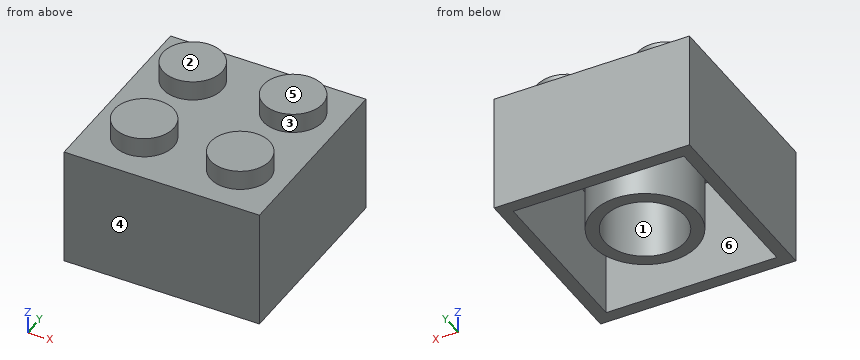
from build123d import *

# Parameters (mm, degrees)
F0_W          = 15.8
F0_H          = 15.8
F1_DEPTH      = 9.6
F4_R          = 2.4
F6_DEPTH      = 1.6
F5_R          = 2.4
F7_DEPTH      = 1.6
F3_R          = 2.4
F8_DEPTH      = 1.6
F2_R          = 2.4
F9_DEPTH      = 1.6
F10_T         = -1
F11_R         = 4.255
F12_DEPTH     = 8.13
F13_T         = 1
F13_T3_DEPTH  = 10.6
F13_T5_DEPTH  = 15.8
F13_T7_DEPTH  = 15.8
F13_T18_ANGLE = 35.7281901551
F13_T20_ANGLE = 210.9230732258
F13_T22_ANGLE = 74.818128958
F13_T24_ANGLE = 41.9866867229
F13_T28_ANGLE = 82.2344866513


# Not quite as in the source:
# - a shell that OpenCascade refuses in one call is made with other operations: the cavity is built on its own and cut out


with BuildPart() as f1:
    # F0 (on Top) → F1 (new body)
    with BuildSketch(Plane.XY):
        Rectangle(F0_W, F0_H)
    extrude(amount=-F1_DEPTH)

    # F4 (on face) → F6 (join)
    with BuildSketch(Plane.XY):
        with Locations((-3.7834926043, -3.5802270286)):
            Circle(F4_R)
    extrude(amount=F6_DEPTH)

    # F5 (on face) → F7 (join)
    with BuildSketch(Plane.XY):
        with Locations((4.0790652856, -3.737478517)):
            Circle(F5_R)
    extrude(amount=F7_DEPTH)

    # F3 (on face) → F8 (join)
    with BuildSketch(Plane.XY):
        with Locations((4.1130073369, 4.042240791)):
            Circle(F3_R)
    extrude(amount=F8_DEPTH)

    # F2 (on face) + F3 (on face) → F9 (join)
    with BuildSketch(Plane.XY):
        with Locations((-4.0000770241, 4.039389547)):
            Circle(F2_R)
    with BuildSketch(Plane.XY):
        with Locations((4.1130073369, 4.042240791)):
            Circle(F3_R)
    extrude(amount=F9_DEPTH)

    # F10
    f10_openings = [f1.faces().sort_by_distance(p)[0] for p in [
        (0, 0, -9.6),
    ]]
    offset(amount=F10_T, openings=f10_openings, kind=Kind.INTERSECTION)

    # F11 (on face) → F12 (join)
    with BuildSketch(Plane(origin=(0, 0, -1), x_dir=(1, 0, 0), z_dir=(0, 0, -1))):
        Circle(F11_R)
    extrude(amount=F12_DEPTH)

    # F13: shell of thickness 1, made by hand


with BuildPart() as f13_core1:
    # F13_t2: copy of F1
    add(f1.part)

    # the walls: a layer under each face that stays
    f13_faces = [f13_core1.faces().sort_by_distance(p)[0] for p in [
        (7.9, 0, -4.8),
        (0, -7.9, -4.8),
        (0, 7.9, -4.8),
        (0, 0, 0),
        (-7.3733333333, -7.3733333333, -9.6),
        (-7.9, 0, -4.8),
        (-6.1834926043, -3.5802270286, 0.8),
        (1.6790652856, -3.737478517, 0.8),
        (-6.4000770241, 4.039389547, 0.8),
        (1.7130073369, 4.042240791, 0.8),
        (6.9, 0, -5.3),
        (0, -6.9, -5.3),
        (-6.9, 0, -5.3),
        (0, 6.9, -5.3),
        (-3.7834926043, -3.5802270286, 1.6),
        (4.0790652856, -3.737478517, 1.6),
        (-4.0000770241, 4.039389547, 1.6),
        (4.1130073369, 4.042240791, 1.6),
        (-4.6, 0, -1),
        (2.6790652856, -3.737478517, -0.2),
        (-4.255, 0, -5.065),
        (-5.1834926043, -3.5802270286, -0.2),
        (-5.4000770241, 4.039389547, -0.2),
        (2.7130073369, 4.042240791, -0.2),
        (3.1153566982, -2.8544722668, -1),
        (4.0790652856, -3.737478517, 0.6),
        (-3.0174039644, -2.8552959816, -1),
        (-3.7834926043, -3.5802270286, 0.6),
        (-4.0000770241, 4.039389547, 0.6),
        (4.1130073369, 4.042240791, 0.6),
    ]]
    thicken(f13_faces, amount=-F13_T, mode=Mode.SUBTRACT)

    # F13_s4 → F13_t3 (cut)
    with BuildSketch(Plane.XY.offset(-10.6)):
        Polygon((6.89, -6.89), (7.9, -6.9), (7.9, -7.9), (6.9, -7.9), align=None)
        Polygon((6.89, 6.89), (7.9, 6.9), (7.9, 7.9), (6.9, 7.9), align=None)
        Polygon((-6.89, -6.89), (-6.9, -7.9), (-7.9, -7.9), (-7.9, -6.9), align=None)
        Polygon((-6.89, 6.89), (-7.9, 6.9), (-7.9, 7.9), (-6.9, 7.9), align=None)
    extrude(amount=F13_T3_DEPTH, mode=Mode.SUBTRACT)

    # F13_s6 → F13_t5 (cut)
    with BuildSketch(Plane.XZ.offset(-7.9)):
        Polygon((6.89, -1.01), (7.9, -1), (7.9, 0), (6.9, 0), align=None)
        Polygon((-6.89, -1.01), (-7.9, -1), (-7.9, 0), (-6.9, 0), align=None)
    extrude(amount=F13_T5_DEPTH, mode=Mode.SUBTRACT)

    # F13_s8 → F13_t7 (cut)
    with BuildSketch(Plane.YZ.offset(-7.9)):
        Polygon((-6.89, -1.01), (-7.9, -1), (-7.9, 0), (-6.9, 0), align=None)
        Polygon((6.89, -1.01), (7.9, -1), (7.9, 0), (6.9, 0), align=None)
    extrude(amount=F13_T7_DEPTH, mode=Mode.SUBTRACT)

    # F13_s9 → F13_t10 (revolve, cut)
    with BuildSketch(Plane.XZ.offset(3.5802270286)):
        Polygon((-1.3734926043, 0.01), (-1.3834926043, -1), (-2.3834926043, -1), (-2.3834926043, 0), align=None)
    revolve(axis=Axis((-3.7834926043, -3.5802270286, 0), (0, 0, 1)), mode=Mode.SUBTRACT)

    # F13_s11 → F13_t12 (revolve, cut)
    with BuildSketch(Plane.XZ.offset(3.737478517)):
        Polygon((6.4890652856, 0.01), (6.4790652856, -1), (5.4790652856, -1), (5.4790652856, 0), align=None)
    revolve(axis=Axis((4.0790652856, -3.737478517, 0), (0, 0, 1)), mode=Mode.SUBTRACT)

    # F13_s13 → F13_t14 (revolve, cut)
    with BuildSketch(Plane.XZ.offset(-4.039389547)):
        Polygon((-1.5900770241, 0.01), (-1.6000770241, -1), (-2.6000770241, -1), (-2.6000770241, 0), align=None)
    revolve(axis=Axis((-4.0000770241, 4.039389547, 0), (0, 0, 1)), mode=Mode.SUBTRACT)

    # F13_s15 → F13_t16 (revolve, cut)
    with BuildSketch(Plane.XZ.offset(-4.042240791)):
        Polygon((6.5230073369, 0.01), (6.5130073369, -1), (5.5130073369, -1), (5.5130073369, 0), align=None)
    revolve(axis=Axis((4.1130073369, 4.042240791, 0), (0, 0, 1)), mode=Mode.SUBTRACT)

    # F13_s17 → F13_t18 (revolve, cut)
    with BuildSketch(Plane.XZ):
        Polygon((4.265, -1.01), (4.255, 0), (3.255, 0), (3.255, -1), align=None)
    revolve(axis=Axis((0, 0, -1), (0, 0, -1)), revolution_arc=F13_T18_ANGLE, mode=Mode.SUBTRACT)

    # F13_s19 → F13_t20 (revolve, cut)
    with BuildSketch(Plane(origin=(0, 0, 0), x_dir=(0, 0, 1), z_dir=(0.5138867564, -0.8578580312, 0))):
        Polygon((-1.01, 4.265), (0, 4.255), (0, 3.255), (-1, 3.255), align=None)
    revolve(axis=Axis((0, 0, -1), (0, 0, -1)), revolution_arc=F13_T20_ANGLE, mode=Mode.SUBTRACT)

    # F13_s21 → F13_t22 (revolve, cut)
    with BuildSketch(Plane(origin=(0, 0, 0), x_dir=(0, 0, 1), z_dir=(0.7577618984, 0.6525311528, 0))):
        Polygon((-1.01, 4.265), (0, 4.255), (0, 3.255), (-1, 3.255), align=None)
    revolve(axis=Axis((0, 0, -1), (0, 0, -1)), revolution_arc=F13_T22_ANGLE, mode=Mode.SUBTRACT)

    # F13_s23 → F13_t24 (revolve, cut)
    with BuildSketch(Plane(origin=(-0.7265604619, -1.8440663308, 0), x_dir=(0, 0, 1), z_dir=(-0.3665725996, -0.9303894503, 0))):
        Polygon((-0.99, -3.7751765248), (-1, -2.7651765248), (-2, -2.7651765248), (-2, -3.7651765248), align=None)
    revolve(axis=Axis((4.0790652856, -3.737478517, -1), (0, 0, -1)), revolution_arc=F13_T24_ANGLE, mode=Mode.SUBTRACT)

    # F13_s25 → F13_t26 (revolve, cut)
    with BuildSketch(Plane.XZ.offset(3.737478517)):
        Polygon((5.4690652856, 0.59), (6.4790652856, 0.6), (6.4790652856, 1.6), (5.4790652856, 1.6), align=None)
    revolve(axis=Axis((4.0790652856, -3.737478517, 0.6), (0, 0, -1)), mode=Mode.SUBTRACT)

    # F13_s27 → F13_t28 (revolve, cut)
    with BuildSketch(Plane(origin=(-3.4098320419, 0.3261629687, 0), x_dir=(0, 0, 1), z_dir=(-0.9954563431, 0.0952190583, 0))):
        Polygon((-0.99, -2.5342203081), (-1, -1.5242203081), (-2, -1.5242203081), (-2, -2.5242203081), align=None)
    revolve(axis=Axis((-3.7834926043, -3.5802270286, -1), (0, 0, -1)), revolution_arc=F13_T28_ANGLE, mode=Mode.SUBTRACT)

    # F13_s29 → F13_t30 (revolve, cut)
    with BuildSketch(Plane.XZ.offset(3.5802270286)):
        Polygon((-2.3934926043, 0.59), (-1.3834926043, 0.6), (-1.3834926043, 1.6), (-2.3834926043, 1.6), align=None)
    revolve(axis=Axis((-3.7834926043, -3.5802270286, 0.6), (0, 0, -1)), mode=Mode.SUBTRACT)

    # F13_s31 → F13_t32 (revolve, cut)
    with BuildSketch(Plane.XZ.offset(-4.039389547)):
        Polygon((-2.6100770241, 0.59), (-1.6000770241, 0.6), (-1.6000770241, 1.6), (-2.6000770241, 1.6), align=None)
    revolve(axis=Axis((-4.0000770241, 4.039389547, 0.6), (0, 0, -1)), mode=Mode.SUBTRACT)

    # F13_s33 → F13_t34 (revolve, cut)
    with BuildSketch(Plane.XZ.offset(-4.042240791)):
        Polygon((5.5030073369, 0.59), (6.5130073369, 0.6), (6.5130073369, 1.6), (5.5130073369, 1.6), align=None)
    revolve(axis=Axis((4.1130073369, 4.042240791, 0.6), (0, 0, -1)), mode=Mode.SUBTRACT)


with BuildPart() as f1_1:
    add(f1.part)

    # what is left inside the walls is the cavity
    f13_cavity = [f13_core1.part.solids().sort_by_distance(p)[0] for p in [
        (-3.245, 0, -6.42),
    ]]
    add(f13_cavity, mode=Mode.SUBTRACT)


solid = f1_1.part
Read the model definition and answer for the solid it produces. Units are mm, in the model's axes. Face numbers are marked on the shaded views. A direction names the side the tool comes from. Coordinates: 2 decimals unless noted, no trailing zeros. Order: outer loops, then holes, each group sorted by start corner. A loop starts at its lowest first (then second) coordinate and runs counter-clockwise, first axis right, second up. Notation, with made-up numbers: M -29.5,66.5 L -14.5,66.5 A24 ccw -14.5,95.5 Z; hole C -15.5,-12 d10. An arc over 180 degrees is marked long. Put each result on its own line as item: value. Start each with the question number.
Item 1: Consider probe 1 along X at (y, z) = (-6.75, -8.75); probe 2 along Y at (x, z) = (-1.75, -7.5). Determine where each line is inside the solid, lowest interval first. Write a range as [from, to].
Item 2: For the marked faces 1, 2 and 3, determine the directions among +Z, -Z, +X, -X, +Y, -Y from which every point of the face is accessible in a straight line to the end or side of a thin tool.
Item 3: Section D-D, the plane z = -8.5 is taken. Determine the outline of the cut face in (x, y) (3 decimals).
Item 4: Given pin 1 Ø3.5 at (x, y) = (-4, 4.04) entering from -Z; pin 2 Ø2 at (x, y) = (-4.5, 4.5) entering from -Z; pin 3 Ø2.5 at (x, y) = (4.11, 4.04) entering from -Z, each flat-ended and moving along its own axis, determine where each tip first touches the part or whether it passes through.
Item 5: Section B-B, the plane y = 0 is taken. Determine the outline of the cut face in (x, z) (3 decimals), plus the area to 3 significant figures.
Item 6: Section A-A, the plane z = -1.25 is taken. Determine the outline of the cut face in (x, y) (1 decimal), plus the area to 3 significant figures.
Item 7: The mould has two halves that part along Y. Classify the marked faces 4, 5 and 6: +Y half, -Y half, draft (parallel to the pull), parting line (faces both ways), or undercut.
Computed:
1. probe 1: x = [-7.9, -6.9], [6.9, 7.9]
1. probe 2: y = [-7.9, -6.9], [-3.88, -2.74], [2.74, 3.88], [6.9, 7.9]
2. face 1: -Z
2. face 2: +Z, +X, -X, +Y, -Y
2. face 3: +Z
3. outline: M -7.9,-7.9 L 7.9,-7.9 L 7.9,7.9 L -7.9,7.9 Z; C 0,0 d8.51; hole M -6.9,-6.9 L 6.9,-6.9 L 6.9,6.9 L -6.9,6.9 Z; hole C 0,0 d6.51
4. pin 1: stops at z = -9.13
4. pin 2: stops at z = -1
4. pin 3: stops at z = 0.6
5. outline: M -7.9,-9.6 L -6.9,-9.6 L -6.9,-1 L -4.255,-1 L -4.255,-9.13 L -3.255,-9.13 L -3.255,-1 L 3.255,-1 L 3.255,-9.13 L 4.255,-9.13 L 4.255,-1 L 6.9,-1 L 6.9,-9.6 L 7.9,-9.6 L 7.9,0 L -7.9,0 Z
5. area: 49.3 mm2
6. outline: M -7.9,-7.9 L 7.9,-7.9 L 7.9,7.9 L -7.9,7.9 Z; C 0,0 d8.5; hole M -6.9,-6.9 L 6.9,-6.9 L 6.9,6.9 L -6.9,6.9 Z; hole M -3,-1.3 A2.4 cw -1.5,-2.9 A3.3 ccw 2,-2.6 A2.4 cw 2.8,-1.7 A3.3 ccw long Z
6. area: 83.5 mm2
7. face 4: -Y half
7. face 5: draft
7. face 6: undercut
